Verification items for the finished model (mm, model axes). A direction names the side the tool comes from. Give positions to 0.01 mm unless a question says otherwise; leave off trailing zeros. Order: outer loops, then holes, each group sorted by start corner. A loop starts at its lowest first (then second) coordinate and runs counter-clockwise, first axis right, second up.
(1) Sectioned sample at C-C on x = 20.5. Record the cut outline in (y, z).
(2) Sectioned sample at A-A on y = 29. Record the cut outline in (x, z).
(3) Sectioned sample at B-B on z = 1.05. Record the cut outline in (x, y).
(4) Mould release check, pull along Y, two halves, no side actions. Record for faces 1 (the face through (181.95, 30, 2)), 2 (the face through (14, 0, 2)), 3 (the face through (27.5, -2, 2)): pulls with the +Y half, pulls with the -Y half, needs draft (parallel to the pull), parting line crosses it, or undercut.
(5) Gauge pin test, flat ends, axial feed: pin 1 (3 mm diameter, centred on x = 123, y = 26.5, fed in from -Z); pin 2 (1 mm diameter, centred on x = 180, z = 2.5, fed in from -Y); pin 3 (1 mm diameter, centred on y = -2, z = 1.5, fed in from -X); pin 4 (1 mm diameter, centred on y = -1.5, z = 2, fed in from +X). Record the tip position at first contact, or that the pin passes through.
(6) Access from +Z, -Z, +X, -X, +Y, -Y to the whole of each face (thin tool, end or side, straight path). Record for faces 4 (the face through (6.95, 30, 2)), 5 (the face through (171, 0, 2)), 6 (the face through (57.5, -2, 2)).
(7) Scan lines: L1, parallel to X at y = 45, z = 0.5; L2, parallel to Y at x = 18.5, z = 1.25. Record each from-to range of solid material in increasing order.
```python
from build123d import *

# Parameters (mm, degrees)
SKETCH_1_W      = 185
SKETCH_1_H      = 60
SKETCH_1_W_2    = 3.9
SKETCH_1_H_2    = 30.4
SKETCH_1_W_3    = 30
SKETCH_1_H_3    = 3.5
EXTRUDE_1_DEPTH = 3.5


with BuildPart() as part:
    # Эскиз1 → Бобышка-Вытянуть1 (new body)
    # profile 1 of 3: a face of its own
    with BuildSketch(Plane.XY):
        with Locations((92.5, 30)):
            Rectangle(SKETCH_1_W, SKETCH_1_H)
        with Locations((180, 30)):
            Rectangle(SKETCH_1_W_2, SKETCH_1_H_2, mode=Mode.SUBTRACT)
        with Locations((5, 30)):
            Rectangle(SKETCH_1_W_2, SKETCH_1_H_2, mode=Mode.SUBTRACT)
    # profile 2 of 3: a face of its own
    with BuildSketch(Plane.XY):
        with Locations((42.5, -1.75)):
            Rectangle(SKETCH_1_W_3, SKETCH_1_H_3)
    # profile 3 of 3: a face of its own
    with BuildSketch(Plane.XY):
        with Locations((142.5, -1.75)):
            Rectangle(SKETCH_1_W_3, SKETCH_1_H_3)
    extrude(amount=EXTRUDE_1_DEPTH)


solid = part.part
```
Ans:
1. outline: (0, 0) - (60, 0) - (60, 3.5) - (0, 3.5) - close
2. outline: (0, 0) - (3.05, 0) - (3.05, 3.5) - (0, 3.5) - close; (6.95, 0) - (178.05, 0) - (178.05, 3.5) - (6.95, 3.5) - close; (181.95, 0) - (185, 0) - (185, 3.5) - (181.95, 3.5) - close
3. outline: (0, 0) - (27.5, 0) - (27.5, -3.5) - (57.5, -3.5) - (57.5, 0) - (127.5, 0) - (127.5, -3.5) - (157.5, -3.5) - (157.5, 0) - (185, 0) - (185, 60) - (0, 60) - close; hole (3.05, 14.8) - (6.95, 14.8) - (6.95, 45.2) - (3.05, 45.2) - close; hole (178.05, 14.8) - (181.95, 14.8) - (181.95, 45.2) - (178.05, 45.2) - close
4. face 1: undercut
4. face 2: pulls with the -Y half
4. face 3: needs draft
5. pin 1: stops at z = 0
5. pin 2: stops at y = 0
5. pin 3: stops at x = 27.5
5. pin 4: stops at x = 157.5
6. face 4: +Z, -Z
6. face 5: +Z, -Z, +X, -Y
6. face 6: +Z, -Z, -Y
7. L1: x = 0 to 3.05, 6.95 to 178.05, 181.95 to 185
7. L2: y = 0 to 60
